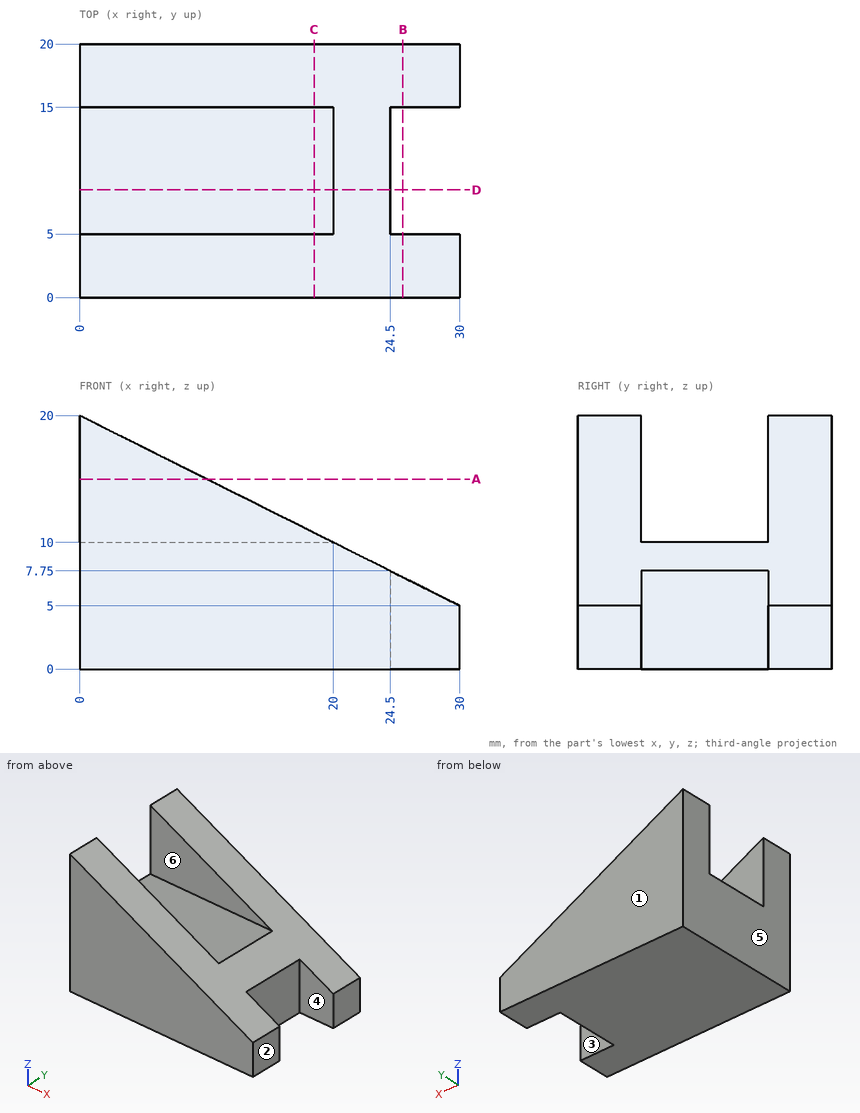
Geometry: see drawing. Coordinates: mm, zero at the bounding-box minimum. A direction names the side the tool comes from. Coordinates: 2 decimals unless noted, no trailing zeros. Loops run counter-clockwise (first coordinate to the right, second up) from the corner with the lowest first, then second, coordinate; pieces in that order, holes last. Notation, with made-up numbers: (60, 73.5) - (85, 73.5) arc R10 cw to (85, 91.5) - close; hole circle Ø7 at (-17, 85.25). An arc over 180 degrees is marked (long way). Put each result on its own line as item: value. Start each with the question number.
Q1. Cut plane B-B, the plane x = 25.5. Return loops of the section in (y, z).
Q2. Pull-direction query (Y, two-part tool) for the marked faces 1, 2 and 3; classes: released by +Y, released by -Y, zero draft, split by the parting line, or undercut.
Q3. Set-up query: the marked faces 4, 5 and 6. Return all of +Z, -Z, +X, -X, +Y, -Y with unobstructed straight access to the full face (end or side cutting, diameter ignored); none if empty.
Q4. Cut plane A-A, the plane z = 15. Return loops of the section in (x, y).
Q5. Cut plane D-D, the plane y = 8.5. Return loops of the section in (x, z).
Q6. Line query: line 1 (Y direction, x = 6, z = 10.25); line 2 (Z direction, x = 7.5, y = 10.25); line 3 (Z direction, x = 23, y = 14). Output: solid intervals per line, ascending.
Q7. Pin query (flat end, axial travel): pin 1 Ø12 at (x, y) = (12, 3) entering from +Z; pin 2 Ø4 at (y, z) = (8, 4.5) entering from +X; pin 3 Ø2 at (x, y) = (17.5, 2.5) entering from +Z. Return the tip coordinate at first contact, or that it passes through.
Q8. Cut plane C-C, the plane x = 18.5. Return loops of the section in (y, z), and give its area (4 significant figures).
Filled sheet:
1. outline: (0, 0) - (5, 0) - (5, 7.25) - (0, 7.25) - close; (15, 0) - (20, 0) - (20, 7.25) - (15, 7.25) - close
2. face 1: released by +Y
2. face 2: zero draft
2. face 3: undercut
3. face 4: +Z, -Z, +X
3. face 5: +Z, -Z, -X, +Y, -Y
3. face 6: +Z, +X, -X
4. outline: (0, 0) - (10, 0) - (10, 5) - (0, 5) - close; (0, 15) - (10, 15) - (10, 20) - (0, 20) - close
5. outline: (0, 0) - (24.5, 0) - (24.5, 7.75) - (20, 10) - (0, 10) - close
6. line 1: 0 to 5, 15 to 20
6. line 2: 0 to 10
6. line 3: 0 to 8.5
7. pin 1: z = 17
7. pin 2: x = 24.5
7. pin 3: z = 11.75
8. outline: (0, 0) - (20, 0) - (20, 10.75) - (15, 10.75) - (15, 10) - (5, 10) - (5, 10.75) - (0, 10.75) - close
8. area: 207.5 mm²
